```python
from build123d import *

# Parameters (mm, degrees)
F0_R        = 1
F0_R_2      = 7
F1_DEPTH    = 6.35
F2_T1_DEPTH = 6.35
F3_R        = 1.995
F4_DEPTH    = 4.35
F5_R        = 2
F6_DEPTH    = 10
F7_R        = 2
F8_DEPTH    = 10


# Not quite as in the source:
# - a fillet or chamfer that OpenCascade refuses, or shapes differently, is made with other operations: its cross-section is extruded or revolved along the edge and cut away or added


with BuildPart() as f1:
    # F0 (on Right) → F1 (new body)
    with BuildSketch(Plane.YZ):
        with BuildLine():
            ThreePointArc((-11, 11.5), (-8.5663313628, 10.4710489148), (-6.4168428396, 8.9344349554))
            ThreePointArc((-6.4168428396, 8.9344349554), (-11, 0), (-6.4168428396, -8.9344349554))
            ThreePointArc((-6.4168428396, -8.9344349554), (-8.5663313628, -10.4710489148), (-11, -11.5))
            Line((-11, -11.5), (-11, -17.5))
            Line((-11, -17.5), (11, -17.5))
            Line((11, -17.5), (11, -11.5))
            ThreePointArc((11, -11.5), (8.5663313628, -10.4710489148), (6.4168428396, -8.9344349554))
            ThreePointArc((6.4168428396, -8.9344349554), (11, 0), (6.4168428396, 8.9344349554))
            ThreePointArc((6.4168428396, 8.9344349554), (8.5663313628, 10.4710489148), (11, 11.5))
            Line((11, 11.5), (11, 17.5))
            Line((11, 17.5), (-11, 17.5))
            Line((-11, 17.5), (-11, 11.5))
        make_face()
        with Locations((0, -9)):
            Circle(F0_R, mode=Mode.SUBTRACT)
        with Locations((-9, 0)):
            Circle(F0_R, mode=Mode.SUBTRACT)
        Circle(F0_R_2, mode=Mode.SUBTRACT)
        with Locations((9, 0)):
            Circle(F0_R, mode=Mode.SUBTRACT)
        with Locations((0, 9)):
            Circle(F0_R, mode=Mode.SUBTRACT)
    extrude(amount=F1_DEPTH)

    # F2: fillet of radius 4 on 4 edges, made by hand

    # F2_s2 → F2_t1 (join)
    with BuildSketch(Plane.YZ):
        with BuildLine():
            ThreePointArc((-10.9998249992, 11.500359687), (-8.9067871665, 9.0142668997), (-9.3494629478, 5.7947167962))
            Line((-9.3494629478, 5.7947167962), (-9.0093791138, 5.5839357582))
            ThreePointArc((-9.0093791138, 5.5839357582), (-7.7456923262, 7.2361578693), (-6.1834406461, 8.6094594545))
            Line((-6.1834406461, 8.6094594545), (-6.1497385524, 9.2323291646))
            ThreePointArc((-6.1497385524, 9.2323291646), (-8.3709064916, 10.8201832442), (-10.8247773704, 11.8601429381))
            Line((-10.8247773704, 11.8601429381), (-10.9998249992, 11.500359687))
        make_face()
        with BuildLine():
            ThreePointArc((-9.3494629478, -5.7947167962), (-8.9067871665, -9.0142668997), (-10.9998249992, -11.500359687))
            Line((-10.9998249992, -11.500359687), (-10.8247773704, -11.8601429381))
            ThreePointArc((-10.8247773704, -11.8601429381), (-8.3709064916, -10.8201832442), (-6.1497385524, -9.2323291646))
            Line((-6.1497385524, -9.2323291646), (-6.1834406461, -8.6094594545))
            ThreePointArc((-6.1834406461, -8.6094594545), (-7.7456923262, -7.2361578693), (-9.0093791138, -5.5839357582))
            Line((-9.0093791138, -5.5839357582), (-9.3494629478, -5.7947167962))
        make_face()
        with BuildLine():
            ThreePointArc((10.9998249992, -11.500359687), (8.9067871665, -9.0142668997), (9.3494629478, -5.7947167962))
            Line((9.3494629478, -5.7947167962), (9.0093791138, -5.5839357582))
            ThreePointArc((9.0093791138, -5.5839357582), (7.7456923262, -7.2361578693), (6.1834406461, -8.6094594545))
            Line((6.1834406461, -8.6094594545), (6.1497385524, -9.2323291646))
            ThreePointArc((6.1497385524, -9.2323291646), (8.3709064916, -10.8201832442), (10.8247773704, -11.8601429381))
            Line((10.8247773704, -11.8601429381), (10.9998249992, -11.500359687))
        make_face()
        with BuildLine():
            ThreePointArc((10.9998249992, 11.500359687), (8.9067871665, 9.0142668997), (9.3494629478, 5.7947167962))
            Line((9.3494629478, 5.7947167962), (9.0093791138, 5.5839357582))
            ThreePointArc((9.0093791138, 5.5839357582), (7.7456923262, 7.2361578693), (6.1834406461, 8.6094594545))
            Line((6.1834406461, 8.6094594545), (6.1497385524, 9.2323291646))
            ThreePointArc((6.1497385524, 9.2323291646), (8.3709064916, 10.8201832442), (10.8247773704, 11.8601429381))
            Line((10.8247773704, 11.8601429381), (10.9998249992, 11.500359687))
        make_face()
    extrude(amount=F2_T1_DEPTH)

    # F3 (on face) → F4 (cut)
    with BuildSketch(Plane.YZ.offset(6.35)):
        with Locations((0, 9)):
            Circle(F3_R)
        with Locations((9, 0)):
            Circle(F3_R)
        with Locations((0, -9)):
            Circle(F3_R)
        with Locations((-9, 0)):
            Circle(F3_R)
    extrude(amount=-F4_DEPTH, mode=Mode.SUBTRACT)

    # F5 (on face) → F6 (cut)
    with BuildSketch(Plane.XY.offset(17.5)):
        with Locations((3.175, 8)):
            Circle(F5_R)
        with Locations((3.175, -8)):
            Circle(F5_R)
    extrude(amount=-F6_DEPTH, mode=Mode.SUBTRACT)

    # F7 (on face) → F8 (cut)
    with BuildSketch(Plane(origin=(0, 0, -17.5), x_dir=(1, 0, 0), z_dir=(0, 0, -1))):
        with Locations((3.175, 8)):
            Circle(F7_R)
        with Locations((3.175, -8)):
            Circle(F7_R)
    extrude(amount=-F8_DEPTH, mode=Mode.SUBTRACT)


solid = f1.part
```
Read the model definition and answer for the solid it produces. Units are mm, in the model's axes. A direction names the side the tool comes from. Coordinates: 2 decimals unless noted, no trailing zeros. Order: outer loops, then holes, each group sorted by start corner. A loop starts at its lowest first (then second) coordinate and runs counter-clockwise, first axis right, second up. Notation, with made-up numbers: (9, 5.5) - (47, 5.5) arc R29 cw to (47, 42.5) - close; hole circle Ø1 at (1.25, 20). An arc over 180 degrees is marked (long way). Answer as a JSON object with one key per item and string values. Group by question number.
Item 1: Section A-A (y = 0) is taken. Give the vertices of the cut face in (x, z) (3 decimals).
Item 2: Section C-C (y = -5) is taken. Give the vertices of the cut face in (x, z).
Item 3: A tool of negligible diameter and unlimited length cuts with its end or side. For faces 1 (the face through (2, -8, -1)), 2 (the face through (2.915, -6.017, 12.57)), 3 (the face through (2.741, -6.048, -12.57)), from which of +Z, -Z, +X, -X, +Y, -Y can it reach the whole face along a straight path? Write none if from no direction.
Item 4: Section D-D (x = 3) is taken. State how many separate pieces and enclosed holes the cut face has, plus the area to 3 significant figures.
Item 5: Section B-B (z = -9) is taken. Give the vertices of the cut face in (x, y) (3 decimals).
Item 6: Flat-ended cylindrical pins translate along their axes: P1, Ø3.5, axis at x = 3.175, y = -8, coming from the +Z side; P2, Ø2.5, axis at y = 0, z = 9, coming from the +X side; P3, Ø0.8, axis at x = 3, y = 7.5, coming from the -Z side; P4, Ø12.5, axis at y = 0, z = 0, coming from the +X side. Find the tip coordinate at first contact, or state that the pin passes through.
Item 7: Consider probe 1 along Z at (x, y) = (1.75, 0); probe 2 along Z at (x, y) = (4.5, -1.25); probe 3 along Y at (x, z) = (3, 1.5). Determine where each line is inside the solid, lowest interval first. Write a range as from..to.
Item 8: The mould has two halves that part along Y. Classify faces 4 (the face through (3.131, -10.926, -1.278)), 5 (the face through (0, -7.5, 0.2)), 6 (the face through (4.21, 9.92, -1.77)): +Y half, -Y half, draft (parallel to the pull), parting line (faces both ways), or undercut.
Results are:
{
 "1": {"outline": "(0, -17.5) - (6.35, -17.5) - (6.35, -10.995) - (2, -10.995) - (2, -10) - (0, -10) - close; (0, -8) - (2, -8) - (2, -7.005) - (6.35, -7.005) - (6.35, -7) - (0, -7) - close; (0, 7) - (6.35, 7) - (6.35, 7.005) - (2, 7.005) - (2, 8) - (0, 8) - close; (0, 10) - (2, 10) - (2, 10.995) - (6.35, 10.995) - (6.35, 17.5) - (0, 17.5) - close"},
 "2": {"outline": "(0, -17.5) - (6.35, -17.5) - (6.35, -4.9) - (0, -4.9) - close; (0, 4.9) - (6.35, 4.9) - (6.35, 17.5) - (0, 17.5) - close"},
 "3": {"face 1": "+X", "face 2": "+Z", "face 3": "-Z"},
 "4": {"separate pieces": "5", "enclosed holes": "5", "area": "366 mm^2"},
 "5": {"outline": "(0, -8.903) - (1.39, -8.903) arc R2 cw (long way) to (4.96, -8.903) - (6.35, -8.903) - (6.35, -1.995) - (2, -1.995) - (2, -1) - (0, -1) - close; (0, 1) - (2, 1) - (2, 1.995) - (6.35, 1.995) - (6.35, 8.903) - (4.96, 8.903) arc R2 cw (long way) to (1.39, 8.903) - (0, 8.903) - close"},
 "6": {"P1": "stops at z = 7.5", "P2": "stops at x = 2", "P3": "stops at z = -7.5", "P4": "passes through"},
 "7": {"probe 1": "z = -17.5..-10, -8..-7, 7..8, 10..17.5", "probe 2": "z = -17.5..-10.55, -7.45..-6.89, 6.89..7.45, 10.55..17.5", "probe 3": "y = -10.9..-10.32, -7.68..-6.84, 6.84..7.68, 10.32..10.9"},
 "8": {"face 4": "-Y half", "face 5": "draft", "face 6": "undercut"}
}
